from build123d import *

# Parameters (mm, degrees)
SKETCH1_R                      = 14.2875
EXTRUDE1_DEPTH                 = 15.24
CUT_EXTRUDE1_DEPTH             = 26.308554137
CUT_EXTRUDE1_DEPTH_BACK        = 26.308554137
TAP_DRILL_FOR_10_TAP1_D        = 4.0386
CHAMFER1_SIZE                  = 0.3937
SKETCH6_R                      = 6.35
CUT_EXTRUDE2_DEPTH             = 0.635
CHAMFER2_SIZE                  = 0.635
CHAMFER3_SIZE                  = 0.381
F_8_6_8_6_DIAMETER_HOLE1_D     = 8.6
F_8_6_8_6_DIAMETER_HOLE1_DEPTH = 15.24
F_8_6_8_6_DIAMETER_HOLE1_TIP   = 2.583700662


with BuildPart() as part:
    # Sketch1 → Extrude1 (new body)
    with BuildSketch(Plane(origin=(0, 0, 0), x_dir=(1, 0, 0), z_dir=(0, 1, 0))):
        with Locations(Location((0, 0, 0), (0, 0, 90))):
            Circle(SKETCH1_R)
    extrude(amount=EXTRUDE1_DEPTH)

    # Sketch3 → Cut-Extrude1 (cut, two sides: drawn at the far end of the back side and taken through both)
    with BuildSketch(Plane(origin=(0, 0, 0), x_dir=(0, 0, -1), z_dir=(1, 0, 0)).offset(-CUT_EXTRUDE1_DEPTH_BACK)):
        Polygon((-10.803384182, 15.24), (10.803384182, 15.24), (2.548384182, 6.985), (-2.548384182, 6.985), align=None)
    extrude(amount=CUT_EXTRUDE1_DEPTH + CUT_EXTRUDE1_DEPTH_BACK, mode=Mode.SUBTRACT)

    # Tap Drill for #10 Tap1 (through all)
    with Locations(Plane.XZ):
        with Locations((-10.16, 0), (10.16, 0)):
            Hole(TAP_DRILL_FOR_10_TAP1_D / 2)

    # Chamfer1
    chamfer1_edges = [part.edges().sort_by_distance(p)[0] for p in [
        (12.1793, 6.985, 0),
        (12.1793, 0, 0),
        (-8.1407, 6.985, 0),
        (-8.1407, 0, 0),
    ]]
    chamfer(chamfer1_edges, length=CHAMFER1_SIZE)

    # Sketch6 → Cut-Extrude2 (cut)
    with BuildSketch(Plane.XZ):
        with Locations(Location((0, 0, 0), (0, 0, 270))):
            Circle(SKETCH6_R)
    extrude(amount=-CUT_EXTRUDE2_DEPTH, mode=Mode.SUBTRACT)

    # Chamfer2
    chamfer2_edges = [part.edges().sort_by_distance(p)[0] for p in [
        (0, 0.635, 6.35),
    ]]
    chamfer(chamfer2_edges, length=CHAMFER2_SIZE - 0.0001)  # a hair under: the kernel refuses the full size

    # Sketch9 → Cut-Revolve1 (revolve, cut)
    with BuildSketch(Plane.XY, mode=Mode.PRIVATE) as cut_revolve1_sk:
        Polygon((2.032, 6.985), (1.5875, 6.5405), (1.5875, 0.9525), (1.905, 0.635), (0, 0.635), (0, 6.985), align=None)
    revolve(cut_revolve1_sk.sketch.rotate(Axis((0, 0, 0), (0, 1, 0)), 90), axis=Axis((0, 0, 0), (0, 1, 0)), mode=Mode.SUBTRACT)

    # Chamfer3
    chamfer3_edges = [part.edges().sort_by_distance(p)[0] for p in [
        (0, 0, 14.2875),
        (4.988953034, 15.24, -13.388166561),
        (0, 15.24, 14.2875),
    ]]
    chamfer(chamfer3_edges, length=CHAMFER3_SIZE)

    # Ø8.6 (8.6) Diameter Hole1
    with Locations(Plane.XZ.offset(-0.635)):
        with Locations((0, 0)):
            Hole(F_8_6_8_6_DIAMETER_HOLE1_D / 2, depth=F_8_6_8_6_DIAMETER_HOLE1_DEPTH)
            with Locations((0, 0, -(F_8_6_8_6_DIAMETER_HOLE1_DEPTH + F_8_6_8_6_DIAMETER_HOLE1_TIP / 2))):  # 118° drill point
                Cone(0, F_8_6_8_6_DIAMETER_HOLE1_D / 2, F_8_6_8_6_DIAMETER_HOLE1_TIP, mode=Mode.SUBTRACT)


solid = part.part
Here's how the part is built. I have some questions about the finished solid (model axes, mm). A direction names the side the tool comes from. Round coordinates to 2 decimals unless told otherwise and drop trailing zeros. Order: outer loops, then holes, each group sorted by start corner. A loop starts at its lowest first (then second) coordinate and runs counter-clockwise, first axis right, second up. Notation, with made-up numbers: M 36,61.5 L 48,61.5 A18 cw 48,83.5 Z; hole C 5,4 d2. An arc over 180 degrees is marked long. One line per question, with ' | ' between items.
1) Imagine slicing it at D-D, the plane y = 11. Write out the boundary of the cut face in (x, z) (1 decimal).
Checked values:
outline: M -12.7,-6.6 A14.3 ccw 12.7,-6.6 Z; M -12.7,6.6 L 12.7,6.6 A14.3 ccw Z
2) I need wall thicknesses on line 1 (Z direction, x = 11.75, y = 5.75); line 2 (Z direction, x = 4.5, y = 7.25); line 3 (Y direction, x = -12.5, z = -0.75) (3 decimals). Which ranges of each line are inside material? Lowest first, please.
Checked values:
line 1: z = -8.13 to -1.24, 1.24 to 8.13 | line 2: z = -13.56 to -2.81, 2.81 to 13.56 | line 3: y = 0 to 6.985
3) I'm going to push flat-ended pins straight in: pin 1 Ø1 at (y, z) = (6, -8.5) entering from -X; pin 2 Ø11 at (x, z) = (0, 0) entering from +Y; pin 3 Ø4.5 at (x, z) = (10.16, 0) entering from -Y; pin 4 Ø4 at (y, z) = (12.5, 3.5) entering from +X. Where does each tip first touch, or does it pass through?
Checked values:
pin 1: stops at x = -11.84 | pin 2: stops at y = 9.94 | pin 3: stops at y = 0.16 | pin 4: passes through
4) Imagine slicing it at A-A, the plane z = 0. Count the separate pieces of the cut face and the enclosed holes in it, plus the area to 3 significant figures.
Checked values:
separate pieces: 4 | enclosed holes: 0 | area: 80.1 mm²
5) We'd pull the mould along Z, two halves only. Please class faces 3 (the flat face through (6, 0, -3)), 4 (the conical face through (-0.148, 15.095, 14.051)), 5 (the flat face through (7.597, 6.985, -0.036)), 6 (the flat face through (4, 0.635, 2)): released by +Z, released by -Z, zero draft, split by the parting line, or undercut.
Checked values:
face 3: zero draft | face 4: released by +Z | face 5: undercut | face 6: undercut
6) Imagine slicing it at C-C, the plane y = 8. Write out the boundary of the cut face in (x, z) (1 decimal), plus the area to 3 significant figures.
Checked values:
outline: M -13.8,-3.6 A14.3 ccw 13.8,-3.6 L 2.4,-3.6 A4.3 cw -2.4,-3.6 Z; M -13.8,3.6 L -2.4,3.6 A4.3 cw 2.4,3.6 L 13.8,3.6 A14.3 ccw Z | area: 435 mm²
7) On a 3-axis mill with a long thin cutter (end or side, diameter ignored), from which of +Z, -Z, +X, -X, +Y, -Y can I reach the whole of each face in a straight line? I mean faces 1 (the flat face through (-0.197, 11.17, -6.734)), 2 (the cylindrical face through (12.177, 3.536, 0.089)). Say none if no direction works.
Checked values:
face 1: +X, -X, +Y | face 2: +Y, -Y
